from build123d import *

# Parameters (mm, degrees)
SKETCH1_W           = 106
SKETCH1_H           = 60
BOSS_EXTRUDE1_DEPTH = 10
SKETCH2_W           = 10
SKETCH2_H           = 60
BOSS_EXTRUDE2_DEPTH = 55
SKETCH3_W           = 30
SKETCH3_H           = 15
BOSS_EXTRUDE3_DEPTH = 20
SKETCH4_W           = 60
SKETCH4_H           = 15
BOSS_EXTRUDE4_DEPTH = 20
SKETCH5_R           = 4.5
CUT_EXTRUDE1_DEPTH  = 66
SKETCH6_R           = 6.5
CUT_EXTRUDE2_DEPTH  = 6.6
SKETCH7_R           = 3.3
CUT_EXTRUDE3_DEPTH  = 9.4
FILLET1_R           = 1


with BuildPart() as part:
    # Sketch1 → Boss-Extrude1 (new body)
    with BuildSketch(Plane(origin=(0, 0, 0), x_dir=(1, 0, 0), z_dir=(0, 1, 0))):
        Rectangle(SKETCH1_W, SKETCH1_H)
    extrude(amount=BOSS_EXTRUDE1_DEPTH)

    # Sketch2 → Boss-Extrude2 (add)
    with BuildSketch(Plane.XZ):
        with Locations((-48, 0)):
            Rectangle(SKETCH2_W, SKETCH2_H)
        with Locations((48, 0)):
            Rectangle(SKETCH2_W, SKETCH2_H)
    extrude(amount=BOSS_EXTRUDE2_DEPTH)

    # Sketch3 → Boss-Extrude3 (add)
    with BuildSketch(Plane(origin=(53, 0, 0), x_dir=(0, 0, -1), z_dir=(1, 0, 0))):
        with Locations((-15, -47.5)):
            Rectangle(SKETCH3_W, SKETCH3_H)
    extrude(amount=BOSS_EXTRUDE3_DEPTH)

    # Sketch4 → Boss-Extrude4 (add)
    with BuildSketch(Plane.ZY.offset(53)):
        with Locations((0, -47.5)):
            Rectangle(SKETCH4_W, SKETCH4_H)
    extrude(amount=BOSS_EXTRUDE4_DEPTH)

    # Sketch5 → Cut-Extrude1 (cut, through all)
    with BuildSketch(Plane(origin=(0, 10, 0), x_dir=(1, 0, 0), z_dir=(0, 1, 0))):
        with Locations((-32, 21)):
            Circle(SKETCH5_R)
        with Locations((32, 21)):
            Circle(SKETCH5_R)
        with Locations((32, -21)):
            Circle(SKETCH5_R)
        with Locations((-32, -21)):
            Circle(SKETCH5_R)
    extrude(amount=-CUT_EXTRUDE1_DEPTH, mode=Mode.SUBTRACT)

    # Sketch6 → Cut-Extrude2 (cut)
    with BuildSketch(Plane(origin=(0, -40, 0), x_dir=(1, 0, 0), z_dir=(0, 1, 0))):
        with Locations((63, -20)):
            Circle(SKETCH6_R)
        with Locations((-63, 20)):
            Circle(SKETCH6_R)
        with Locations((-63, -20)):
            Circle(SKETCH6_R)
    extrude(amount=-CUT_EXTRUDE2_DEPTH, mode=Mode.SUBTRACT)

    # Sketch7 → Cut-Extrude3 (cut, through all)
    with BuildSketch(Plane(origin=(0, -46.6, 0), x_dir=(1, 0, 0), z_dir=(0, 1, 0))):
        with Locations((-63, 20)):
            Circle(SKETCH7_R)
        with Locations((-63, -20)):
            Circle(SKETCH7_R)
        with Locations((63, -20)):
            Circle(SKETCH7_R)
    extrude(amount=-CUT_EXTRUDE3_DEPTH, mode=Mode.SUBTRACT)

    # Fillet1
    fillet1_edges = [part.edges().sort_by_distance(p)[0] for p in [
        (-43, -27.5, -30),
        (-43, -27.5, 30),
        (43, -27.5, 30),
        (43, -27.5, -30),
        (73, -47.5, 30),
        (73, -47.5, 0),
        (-73, -47.5, -30),
        (-73, -47.5, 30),
    ]]
    fillet(fillet1_edges, radius=FILLET1_R)


solid = part.part
The model under review builds one solid part; all positions refer to its coordinate system, in mm. A direction names the side the tool comes from. Give positions to 0.01 mm unless a question says otherwise; leave off trailing zeros. Order: outer loops, then holes, each group sorted by start corner. A loop starts at its lowest first (then second) coordinate and runs counter-clockwise, first axis right, second up. Notation, with made-up numbers: (14, 18.25) -> (43, 18.25) arc R16 ccw to (43, 35.25) -> close; hole circle Ø10 at (78.5, -13). An arc over 180 degrees is marked (long way). Write item = value, one per line. Start each with the question number.
(1) Tool access review of faces 4 (the flat face through (-53, -15, 0)), 5 (the flat face through (43, -27, 0)), 6 (the flat face through (-66, -46.6, -22)), 7 (the flat face through (62, -48, 0)): name each direction out of +Z, -Z, +X, -X, +Y, -Y from which nothing blocks a thin tool from reaching the whole face with its end or side.
(2) Take a section at B-B (y = -22). Write out the cut boundary in (x, z).
(3) For pin 1 Ø10.5 at (x, z) = (-63, -20) entering from +Y; pin 2 Ø6 at (y, z) = (-48.5, -6) entering from +X; pin 3 Ø14.5 at (x, z) = (32, 21) entering from -Y, all flat-tipped, find the tip position at first contact; note any pin that passes through.
(4) Draft analysis for pull direction Z (two halves, no side actions). For faces 1 (the cylindrical face through (-56.8, -43.25, -21.95)), 2 (the flat face through (-10, 1, 30)), 3 (the flat face through (63, -40, 12)), state which applies: +Z half, -Z half, draft (parallel to the pull), parting line (faces both ways), or undercut.
(5) Take a section at A-A (x = 63). Write out the cut boundary in (y, z).
(6) Take a section at C-C (x = -63). Write out the cut boundary in (y, z), plus the area to 3 significant figures.
(7) For L1, parallel to Z at x = -63, y = -45; L2, parallel to X at y = -41.5, z = 20; L3, parallel to X at y = -52.75, z = 20, list the stretches that pass through material, from the lowest coordinate up. Write a range as from..to.
(8) Take a section at D-D (z = -11). Write out the cut boundary in (x, y), plus the area to 3 significant figures.
Returned:
q1.face_4 = +Z, -Z, -X, +Y
q1.face_5 = +Z, -Z, -Y
q1.face_6 = +Y
q1.face_7 = -Z, +X, +Y, -Y
q2.outline = (-53, -30) -> (-44, -30) arc R1 ccw to (-43, -29) -> (-43, 29) arc R1 ccw to (-44, 30) -> (-53, 30) -> close; (43, -29) arc R1 ccw to (44, -30) -> (53, -30) -> (53, 30) -> (44, 30) arc R1 ccw to (43, 29) -> close
q3.pin_1 = -46.6
q3.pin_2 = 53
q3.pin_3 = 0
q4.face_1 = undercut
q4.face_2 = +Z half
q4.face_3 = draft
q5.outline = (-55, 0) -> (-40, 0) -> (-40, 13.5) -> (-46.6, 13.5) -> (-46.6, 16.7) -> (-55, 16.7) -> close; (-55, 23.3) -> (-46.6, 23.3) -> (-46.6, 26.5) -> (-40, 26.5) -> (-40, 30) -> (-55, 30) -> close
q6.outline = (-55, -30) -> (-40, -30) -> (-40, -26.5) -> (-46.6, -26.5) -> (-46.6, -23.3) -> (-55, -23.3) -> close; (-55, -16.7) -> (-46.6, -16.7) -> (-46.6, -13.5) -> (-40, -13.5) -> (-40, 13.5) -> (-46.6, 13.5) -> (-46.6, 16.7) -> (-55, 16.7) -> close; (-55, 23.3) -> (-46.6, 23.3) -> (-46.6, 26.5) -> (-40, 26.5) -> (-40, 30) -> (-55, 30) -> close
q6.area = 618 mm²
q7.L1 = -30..-26.5, -13.5..13.5, 26.5..30
q7.L2 = -73..-69.5, -56.5..-43, 43..56.5, 69.5..73
q7.L3 = -73..-66.3, -59.7..-43, 43..59.7, 66.3..73
q8.outline = (-73, -55) -> (-43, -55) -> (-43, 0) -> (43, 0) -> (43, -55) -> (53, -55) -> (53, 10) -> (-53, 10) -> (-53, -40) -> (-73, -40) -> close
q8.area = 2,460 mm²
